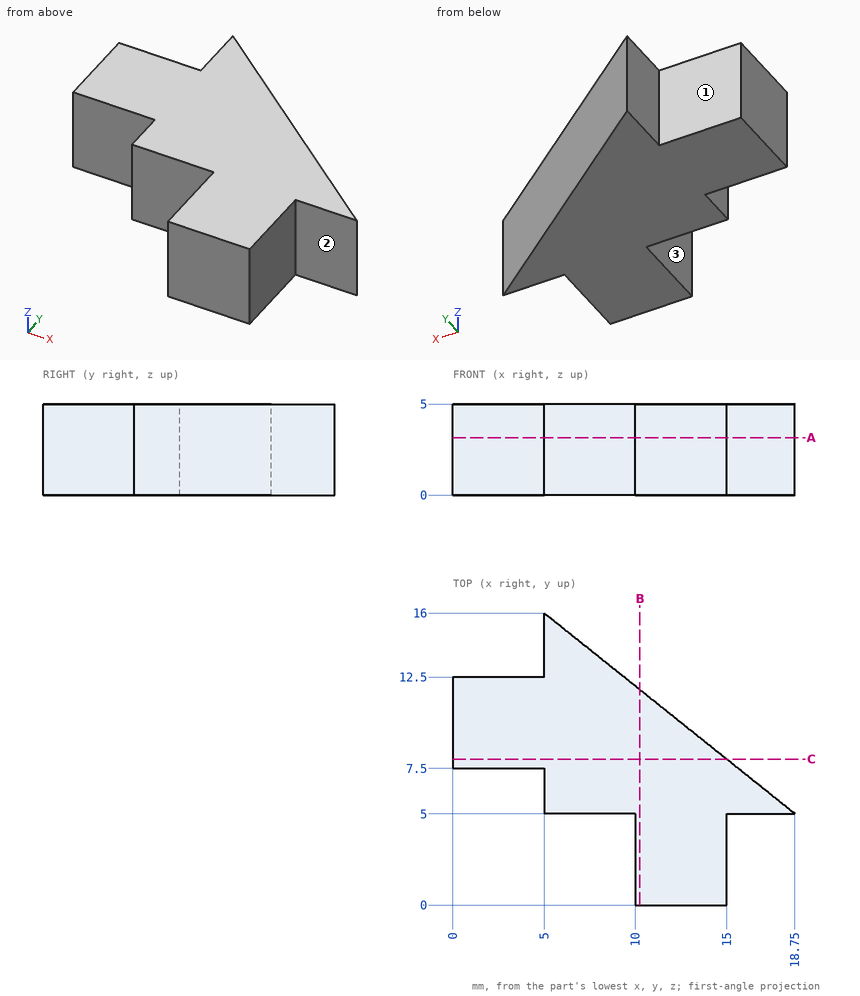
Study the drawing (mm; zero at the part's minimum x, y, z) and answer. A direction names the side the tool comes from. Give positions to 0.01 mm unless a question says otherwise; leave off trailing zeros. Loops run counter-clockwise (first coordinate to the right, second up) from the corner with the lowest first, then second, coordinate; pieces in that order, holes last. Notation, with made-up numbers: (56, 21) - (84, 21) arc R18 ccw to (84, 35) - close; hole circle Ø8 at (3, 27.25). An arc over 180 degrees is marked (long way). Answer as CSV lines item,"result". Start each with the question number.
1) Straight lines are drawn through the part: L1, parallel to X at y = 2.75, z = 1.8; L2, parallel to Y at x = 4.5, z = 0.9; L3, parallel to Y at x = 5.75, z = 3.4. For each, find the intervals that lie inside material, in ascending order. Write a range as from..to.
2) Find section A-A (z = 3.15). Write down the section's boundary in (x, y), then the cut area to 3 significant figures.
3) Find section B-B (x = 10.25). Write down the section's boundary in (y, z).
4) Which of the six approach directions +Z, -Z, +X, -X, +Y, -Y give full straight-line access (tool end or side, diameter ignored) to the marked faces 1, 2 and 3?
5) Find section C-C (y = 8). Write down the section's boundary in (x, z).
6) Each of these flat-tipped pins is pushed along its axis until it touches: pin 1 Ø1.8 at (y, z) = (13.5, 3.5) entering from -X; pin 2 Ø2 at (y, z) = (1.5, 4.5) entering from -X; pin 3 Ø1.5 at (y, z) = (3.5, 2.5) entering from +X; pin 4 Ø5 at (x, y) = (12, 12.5) entering from +Z. Where does it stop, or does it pass through?
Findings below:
1,L1,"10..15"
1,L2,"7.5..12.5"
1,L3,"5..15.4"
2,outline,"(0, 7.5) - (5, 7.5) - (5, 5) - (10, 5) - (10, 0) - (15, 0) - (15, 5) - (18.75, 5) - (5, 16) - (5, 12.5) - (0, 12.5) - close"
2,area,"126 mm^2"
3,outline,"(0, 0) - (11.8, 0) - (11.8, 5) - (0, 5) - close"
4,face 1,"+Z, -Z, -X, +Y"
4,face 2,"+Z, -Z, +X, -Y"
4,face 3,"+Z, -Z, -X, -Y"
5,outline,"(0, 0) - (15, 0) - (15, 5) - (0, 5) - close"
6,pin 1,"x = 5"
6,pin 2,"x = 10"
6,pin 3,"x = 15"
6,pin 4,"z = 5"
